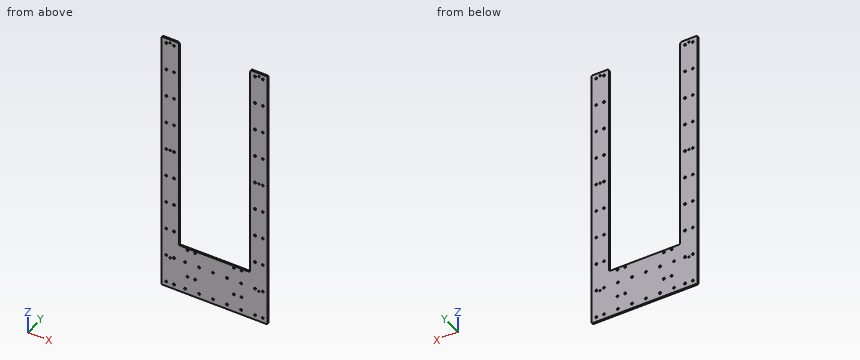
```python
from build123d import *

# Parameters (mm, degrees)
SKETCH1_R           = 2.1
SKETCH1_R_2         = 1.6
BOSS_EXTRUDE1_DEPTH = 3.175
FILLET1_R           = 3.2


with BuildPart() as part:
    # Sketch1 → Boss-Extrude1 (new body)
    with BuildSketch(Plane(origin=(0, 0, 0), x_dir=(1, 0, 0), z_dir=(0, 1, 0))):
        Polygon((-110, -271), (-74, -271), (-74, 171), (74, 171), (74, -271), (110, -271), (110, 271), (-110, 271), align=None)
        with Locations(Location((100, 261, 0), (0, 0, 270))):
            Circle(SKETCH1_R, mode=Mode.SUBTRACT)
        with Locations(Location((100, 203, 0), (0, 0, 270))):
            Circle(SKETCH1_R, mode=Mode.SUBTRACT)
        with Locations(Location((100, 145, 0), (0, 0, 270))):
            Circle(SKETCH1_R, mode=Mode.SUBTRACT)
        with Locations(Location((100, 87, 0), (0, 0, 270))):
            Circle(SKETCH1_R, mode=Mode.SUBTRACT)
        with Locations(Location((100, 29, 0), (0, 0, 270))):
            Circle(SKETCH1_R, mode=Mode.SUBTRACT)
        with Locations(Location((100, -29, 0), (0, 0, 270))):
            Circle(SKETCH1_R, mode=Mode.SUBTRACT)
        with Locations(Location((100, -87, 0), (0, 0, 270))):
            Circle(SKETCH1_R, mode=Mode.SUBTRACT)
        with Locations(Location((100, -145, 0), (0, 0, 270))):
            Circle(SKETCH1_R, mode=Mode.SUBTRACT)
        with Locations(Location((100, -203, 0), (0, 0, 270))):
            Circle(SKETCH1_R, mode=Mode.SUBTRACT)
        with Locations(Location((100, -261, 0), (0, 0, 270))):
            Circle(SKETCH1_R, mode=Mode.SUBTRACT)
        with Locations(Location((84, -261, 0), (0, 0, 270))):
            Circle(SKETCH1_R, mode=Mode.SUBTRACT)
        with Locations(Location((84, -203, 0), (0, 0, 270))):
            Circle(SKETCH1_R, mode=Mode.SUBTRACT)
        with Locations(Location((84, -145, 0), (0, 0, 270))):
            Circle(SKETCH1_R, mode=Mode.SUBTRACT)
        with Locations(Location((84, -87, 0), (0, 0, 270))):
            Circle(SKETCH1_R, mode=Mode.SUBTRACT)
        with Locations(Location((84, -29, 0), (0, 0, 270))):
            Circle(SKETCH1_R, mode=Mode.SUBTRACT)
        with Locations(Location((84, 29, 0), (0, 0, 270))):
            Circle(SKETCH1_R, mode=Mode.SUBTRACT)
        with Locations(Location((84, 87, 0), (0, 0, 270))):
            Circle(SKETCH1_R, mode=Mode.SUBTRACT)
        with Locations(Location((84, 145, 0), (0, 0, 270))):
            Circle(SKETCH1_R, mode=Mode.SUBTRACT)
        with Locations(Location((84, 203, 0), (0, 0, 270))):
            Circle(SKETCH1_R, mode=Mode.SUBTRACT)
        with Locations(Location((84, 261, 0), (0, 0, 270))):
            Circle(SKETCH1_R, mode=Mode.SUBTRACT)
        with Locations(Location((92, -29, 0), (0, 0, 270))):
            Circle(SKETCH1_R_2, mode=Mode.SUBTRACT)
        with Locations(Location((92, 206, 0), (0, 0, 270))):
            Circle(SKETCH1_R_2, mode=Mode.SUBTRACT)
        with Locations(Location((92, -264, 0), (0, 0, 270))):
            Circle(SKETCH1_R_2, mode=Mode.SUBTRACT)
        with Locations(Location((-100, 261, 0), (0, 0, 270))):
            Circle(SKETCH1_R, mode=Mode.SUBTRACT)
        with Locations(Location((-84, 261, 0), (0, 0, 270))):
            Circle(SKETCH1_R, mode=Mode.SUBTRACT)
        with Locations(Location((-92, 206, 0), (0, 0, 270))):
            Circle(SKETCH1_R_2, mode=Mode.SUBTRACT)
        with Locations(Location((-84, 87, 0), (0, 0, 270))):
            Circle(SKETCH1_R, mode=Mode.SUBTRACT)
        with Locations(Location((-100, 87, 0), (0, 0, 270))):
            Circle(SKETCH1_R, mode=Mode.SUBTRACT)
        with Locations(Location((-100, 145, 0), (0, 0, 270))):
            Circle(SKETCH1_R, mode=Mode.SUBTRACT)
        with Locations(Location((-100, 203, 0), (0, 0, 270))):
            Circle(SKETCH1_R, mode=Mode.SUBTRACT)
        with Locations(Location((-92, -264, 0), (0, 0, 270))):
            Circle(SKETCH1_R_2, mode=Mode.SUBTRACT)
        with Locations(Location((-92, -29, 0), (0, 0, 270))):
            Circle(SKETCH1_R_2, mode=Mode.SUBTRACT)
        with Locations(Location((-84, 29, 0), (0, 0, 270))):
            Circle(SKETCH1_R, mode=Mode.SUBTRACT)
        with Locations(Location((-84, -29, 0), (0, 0, 270))):
            Circle(SKETCH1_R, mode=Mode.SUBTRACT)
        with Locations(Location((-84, -87, 0), (0, 0, 270))):
            Circle(SKETCH1_R, mode=Mode.SUBTRACT)
        with Locations(Location((-84, -145, 0), (0, 0, 270))):
            Circle(SKETCH1_R, mode=Mode.SUBTRACT)
        with Locations(Location((-84, -203, 0), (0, 0, 270))):
            Circle(SKETCH1_R, mode=Mode.SUBTRACT)
        with Locations(Location((-84, -261, 0), (0, 0, 270))):
            Circle(SKETCH1_R, mode=Mode.SUBTRACT)
        with Locations(Location((-100, -261, 0), (0, 0, 270))):
            Circle(SKETCH1_R, mode=Mode.SUBTRACT)
        with Locations(Location((-100, -203, 0), (0, 0, 270))):
            Circle(SKETCH1_R, mode=Mode.SUBTRACT)
        with Locations(Location((-100, -145, 0), (0, 0, 270))):
            Circle(SKETCH1_R, mode=Mode.SUBTRACT)
        with Locations(Location((-100, -87, 0), (0, 0, 270))):
            Circle(SKETCH1_R, mode=Mode.SUBTRACT)
        with Locations(Location((-100, -29, 0), (0, 0, 270))):
            Circle(SKETCH1_R, mode=Mode.SUBTRACT)
        with Locations(Location((-100, 29, 0), (0, 0, 270))):
            Circle(SKETCH1_R, mode=Mode.SUBTRACT)
        with Locations(Location((-84, 203, 0), (0, 0, 270))):
            Circle(SKETCH1_R, mode=Mode.SUBTRACT)
        with Locations(Location((-84, 145, 0), (0, 0, 270))):
            Circle(SKETCH1_R, mode=Mode.SUBTRACT)
        with Locations(Location((55, 261, 0), (0, 0, 270))):
            Circle(SKETCH1_R, mode=Mode.SUBTRACT)
        with Locations(Location((26, 261, 0), (0, 0, 270))):
            Circle(SKETCH1_R, mode=Mode.SUBTRACT)
        with Locations(Location((-3, 261, 0), (0, 0, 270))):
            Circle(SKETCH1_R, mode=Mode.SUBTRACT)
        with Locations(Location((-32, 261, 0), (0, 0, 270))):
            Circle(SKETCH1_R, mode=Mode.SUBTRACT)
        with Locations(Location((-61, 261, 0), (0, 0, 270))):
            Circle(SKETCH1_R, mode=Mode.SUBTRACT)
        with Locations(Location((55, 203, 0), (0, 0, 270))):
            Circle(SKETCH1_R, mode=Mode.SUBTRACT)
        with Locations(Location((26, 203, 0), (0, 0, 270))):
            Circle(SKETCH1_R, mode=Mode.SUBTRACT)
        with Locations(Location((-3, 203, 0), (0, 0, 270))):
            Circle(SKETCH1_R, mode=Mode.SUBTRACT)
        with Locations(Location((-32, 203, 0), (0, 0, 270))):
            Circle(SKETCH1_R, mode=Mode.SUBTRACT)
        with Locations(Location((-61, 203, 0), (0, 0, 270))):
            Circle(SKETCH1_R, mode=Mode.SUBTRACT)
        with Locations(Location((-56, 175, 0), (0, 0, 270))):
            Circle(SKETCH1_R, mode=Mode.SUBTRACT)
        with Locations(Location((-40, 175, 0), (0, 0, 270))):
            Circle(SKETCH1_R, mode=Mode.SUBTRACT)
        with Locations(Location((-40, 233, 0), (0, 0, 270))):
            Circle(SKETCH1_R, mode=Mode.SUBTRACT)
        with Locations(Location((-56, 233, 0), (0, 0, 270))):
            Circle(SKETCH1_R, mode=Mode.SUBTRACT)
        with Locations(Location((40, 175, 0), (0, 0, 270))):
            Circle(SKETCH1_R, mode=Mode.SUBTRACT)
        with Locations(Location((56, 175, 0), (0, 0, 270))):
            Circle(SKETCH1_R, mode=Mode.SUBTRACT)
        with Locations(Location((56, 233, 0), (0, 0, 270))):
            Circle(SKETCH1_R, mode=Mode.SUBTRACT)
        with Locations(Location((40, 233, 0), (0, 0, 270))):
            Circle(SKETCH1_R, mode=Mode.SUBTRACT)
    extrude(amount=BOSS_EXTRUDE1_DEPTH)

    # Fillet1
    fillet1_edges = [part.edges().sort_by_distance(p)[0] for p in [
        (74, 1.5875, -171),
        (-74, 1.5875, -171),
        (-74, 1.5875, 271),
        (-110, 1.5875, 271),
        (-110, 1.5875, -271),
        (110, 1.5875, -271),
        (110, 1.5875, 271),
        (74, 1.5875, 271),
    ]]
    fillet(fillet1_edges, radius=FILLET1_R)


solid = part.part
```
Model file for the job. Use its own axes, mm. Give positions to 0.01 mm unless a question says otherwise; leave off trailing zeros. Loops run counter-clockwise (first coordinate to the right, second up) from the corner with the lowest first, then second, coordinate; pieces in that order, holes last. Notation, with made-up numbers: (-1, 43) -> (37, 43) arc R28 ccw to (37, 71) -> close; hole circle Ø11 at (68.5, 80). An arc over 180 degrees is marked (long way). Write each question's results on one line, items separated by ' | '.
(1) Flat gauge pins, fed straight in: pin 1 Ø12 at (x, z) = (69.5, 27.5) entering from +Y (3 decimals); pin 2 Ø2.5 at (x, z) = (-61, -203) entering from +Y. Where does each tip first touch, or does it go through?
Geometry results:
pin 1: stops at y = 3.175 | pin 2: passes through
(2) Probe line 1 along X through (y, z) = (2.25, -206); line 2 along X through (y, z) = (1.9, 87); line 3 along Z through (x, y) = (92, 1). List the from-to ranges inside material, lowest first.
Geometry results:
line 1: x = -110 to -93.6, -90.4 to 90.4, 93.6 to 110 | line 2: x = -110 to -102.1, -97.9 to -86.1, -81.9 to -74, 74 to 81.9, 86.1 to 97.9, 102.1 to 110 | line 3: z = -271 to -207.6, -204.4 to 27.4, 30.6 to 262.4, 265.6 to 271
(3) Cut at B-B on y = 1.55. Give the number of separate pieces and of enclosed holes in the cut face, and give its area (3 significant figures).
Geometry results:
separate pieces: 1 | enclosed holes: 64 | area: 53,000 mm²
(4) Cut at A-A on z = -75.5. List the corners of the cut face in (x, y) (3 decimals).
Geometry results:
outline: (-110, 0) -> (-74, 0) -> (-74, 3.175) -> (-110, 3.175) -> close; (74, 0) -> (110, 0) -> (110, 3.175) -> (74, 3.175) -> close
(5) Cut at C-C on x = 15. List the corners of the cut face in (y, z) (3 decimals), and give its area (4 significant figures).
Geometry results:
outline: (0, -271) -> (3.175, -271) -> (3.175, -171) -> (0, -171) -> close | area: 317.5 mm²
